Verification items for the finished model (mm, model axes). A direction names the side the tool comes from. Coordinates: 2 decimals unless noted, no trailing zeros. Write each loop counter-clockwise with the first axis right and the second up, starting at its lowest first coordinate (ties: lowest second). Pieces come first, ordered by that corner, then holes. Notation, with made-up numbers: (50.25, -10.5) -> (75.25, -10.5) arc R27 cw to (75.25, 27.5) -> close; hole circle Ø3 at (71, 43.25). An arc over 180 degrees is marked (long way). Answer in a Markdown table with one row per item.
Autodesk Fusion 360 part; units mm, degrees
sketch "base" plane through (0, 0, 0) normal (0, 0, 1) x (1, 0, 0) in component "base"
  line L0 (50, 50) -> (-50, 50)
  line L1 (-50, 50) -> (-50, -50)
  line L2 (-50, -50) -> (50, -50)
  line L3 (50, -50) -> (50, 50)
  line L4 (50, 50) -> (-50, -50) construction
  line L5 (-50, 50) -> (50, -50) construction
  dimension "d1" = 100
  dimension "d2" = 100
extrude "Extrude1" add sketch "base" along normal blind 3 in component "base"
sketch "legs" plane through (0, 0, 0) normal (0, 0, -1) x (1, 0, 0) in component "base"
  line L0 (50, -50) -> (50, 50)
  line L1 (50, 50) -> (-50, 50)
  line L2 (-50, 50) -> (-50, -50)
  line L3 (-50, -50) -> (50, -50)
  line L4 (47.5, 47.5) -> (-47.5, 47.5)
  line L5 (-47.5, 47.5) -> (-47.5, -47.5)
  line L6 (-47.5, -47.5) -> (47.5, -47.5)
  line L7 (47.5, -47.5) -> (47.5, 47.5)
  line L8 (47.5, 47.5) -> (-47.5, -47.5) construction
  line L9 (-47.5, 47.5) -> (47.5, -47.5) construction
  line L10 (-50, -50) -> (50, -50)
  line L11 (50, -50) -> (50, 50)
  line L12 (50, 50) -> (-50, 50)
  line L13 (-50, 50) -> (-50, -50)
  dimension "d5" = 95
  dimension "d6" = 95
  dimension "d7" = 2.5
extrude "Extrude2" add sketch "legs" along normal blind 40 in component "base"
component "base" placed x (1, 0, 0) y (0, 1, 0) z (0, 0, 1) at (0, 0, 0)
1. Release check for a two-part mould opening along Y. For faces 1 (the face through (1, -47.5, -20)), 2 (the face through (-50, 1, -19)), 3 (the face through (1, 50, -19)) record: released by +Y, released by -Y, zero draft, split by the parting line, or undercut.
Findings below:
| item | result |
|---|---|
| face 1 | undercut |
| face 2 | zero draft |
| face 3 | released by +Y |
2. Sectioned sample at B-B, the plane z = -13. Record the cut outline in (x, y).
Findings below:
| item | result |
|---|---|
| outline | (-50, -50) -> (50, -50) -> (50, 50) -> (-50, 50) -> close; hole (-47.5, -47.5) -> (47.5, -47.5) -> (47.5, 47.5) -> (-47.5, 47.5) -> close |
3. Go/stop test with a flat-tipped pin: pin 1 (4 mm diameter, centred on x = -32, y = 23.5, fed in from -Z). Record where the tip stops, or that it passes through.
Findings below:
| item | result |
|---|---|
| pin 1 | stops at z = 0 |
4. Sectioned sample at A-A, the plane y = 18.5. Record the cut outline in (x, z).
Findings below:
| item | result |
|---|---|
| outline | (-50, -40) -> (-47.5, -40) -> (-47.5, 0) -> (47.5, 0) -> (47.5, -40) -> (50, -40) -> (50, 3) -> (-50, 3) -> close |
5. Access from +Z, -Z, +X, -X, +Y, -Y to the whole of each face (thin tool, end or side, straight path). Record for faces 4 (the face through (47.5, 1, -20)), 5 (the face through (-4, 48, -40)).
Findings below:
| item | result |
|---|---|
| face 4 | -Z |
| face 5 | -Z, +X, -X, +Y, -Y |
6. Material ranges on probe 1 along Y at (x, z) = (25.5, -32); probe 2 along Z at (x, y) = (36, 45.5), recorded low to high. Write a range as from..to.
Findings below:
| item | result |
|---|---|
| probe 1 | y = -50..-47.5, 47.5..50 |
| probe 2 | z = 0..3 |
